from build123d import *

# Parameters (mm, degrees)
SKETCH1_W           = 85.8
SKETCH1_H           = 92.5
SKETCH1_R           = 2.05
BOSS_EXTRUDE1_DEPTH = 3.175
SKETCH2_W           = 85.8
SKETCH2_H           = 92.5
SKETCH2_R           = 1.35
SKETCH2_R_2         = 3.35
BOSS_EXTRUDE2_DEPTH = 1.905
BOSS_EXTRUDE3_START = 1
SKETCH2_3_W         = 85.8
SKETCH2_3_H         = 92.5
SKETCH2_3_R         = 1.35
SKETCH2_3_R_2       = 3.35
BOSS_EXTRUDE3_DEPTH = 1
SKETCH3_W           = 85.8
SKETCH3_H           = 92.5
SKETCH3_W_2         = 75.8
SKETCH3_H_2         = 82.5
BOSS_EXTRUDE4_DEPTH = 4.55
SKETCH4_W           = 14
SKETCH4_H           = 6.75
CUT_EXTRUDE1_DEPTH  = 118.864146478
SKETCH5_W           = 10
SKETCH5_H           = 6
CUT_EXTRUDE2_DEPTH  = 118.864146478
BOSS_EXTRUDE5_DEPTH = 3.5
FILLET1_R           = 2.5
FILLET2_R           = 2.5
FILLET3_R           = 2.5
FILLET4_R           = 2.5
FILLET5_R           = 2.5
CUT_EXTRUDE3_DEPTH  = 3.36
CUT_EXTRUDE4_DEPTH  = 75
SKETCH10_W          = 4.501
SKETCH10_H          = 3
BOSS_EXTRUDE6_DEPTH = 5


with BuildPart() as part:
    # Sketch1 → Boss-Extrude1 (new body)
    with BuildSketch(Plane(origin=(0, 0, 0), x_dir=(1, 0, 0), z_dir=(0, 1, 0))):
        with Locations((36.9, 40.25)):
            Rectangle(SKETCH1_W, SKETCH1_H)
        with Locations(Location((2.5, 12.5, 0), (0, 0, 270))):
            Circle(SKETCH1_R, mode=Mode.SUBTRACT)
        with Locations(Location((18.4, 2.5, 0), (0, 0, 270))):
            Circle(SKETCH1_R, mode=Mode.SUBTRACT)
        with Locations(Location((36.9, 2.5, 0), (0, 0, 270))):
            Circle(SKETCH1_R, mode=Mode.SUBTRACT)
        with Locations(Location((55.4, 2.5, 0), (0, 0, 270))):
            Circle(SKETCH1_R, mode=Mode.SUBTRACT)
        with Locations(Location((29.3, 55.1, 0), (0, 0, 270))):
            Circle(SKETCH1_R, mode=Mode.SUBTRACT)
        with Locations(Location((70.8, 74.5, 0), (0, 0, 270))):
            Circle(SKETCH1_R, mode=Mode.SUBTRACT)
    extrude(amount=BOSS_EXTRUDE1_DEPTH)

    # Sketch2 → Boss-Extrude2 (add)
    # profile 1 of 2: a face of its own
    with BuildSketch(Plane(origin=(0, 0, 0), x_dir=(1, 0, 0), z_dir=(0, 1, 0))):
        with Locations((36.9, 40.25)):
            Rectangle(SKETCH2_W, SKETCH2_H)
        with Locations(Location((2.5, 12.5, 0), (0, 0, 270))):
            Circle(SKETCH2_R, mode=Mode.SUBTRACT)
        with Locations(Location((18.4, 2.5, 0), (0, 0, 270))):
            Circle(SKETCH2_R, mode=Mode.SUBTRACT)
        with Locations(Location((36.9, 2.5, 0), (0, 0, 270))):
            Circle(SKETCH2_R, mode=Mode.SUBTRACT)
        with Locations(Location((55.4, 2.5, 0), (0, 0, 270))):
            Circle(SKETCH2_R, mode=Mode.SUBTRACT)
        with Locations(Location((70.8, 74.5, 0), (0, 0, 270))):
            Circle(SKETCH2_R, mode=Mode.SUBTRACT)
        with BuildLine():
            Line((65.8, 74.5), (65.8, 81.5))
            Line((65.8, 81.5), (-1, 81.5))
            Line((-1, 81.5), (-1, 17.5))
            Line((-1, 17.5), (2.5, 17.5))
            ThreePointArc((2.5, 17.5), (7.5, 12.5), (2.5, 7.5))
            Line((2.5, 7.5), (-1, 7.5))
            Line((-1, 7.5), (-1, -1))
            Line((-1, -1), (13.4, -1))
            Line((13.4, -1), (13.4, 2.5))
            ThreePointArc((13.4, 2.5), (18.4, 7.5), (23.4, 2.5))
            Line((23.4, 2.5), (23.4, -1))
            Line((23.4, -1), (31.9, -1))
            Line((31.9, -1), (31.9, 2.5))
            ThreePointArc((31.9, 2.5), (36.9, 7.5), (41.9, 2.5))
            Line((41.9, 2.5), (41.9, -1))
            Line((41.9, -1), (50.4, -1))
            Line((50.4, -1), (50.4, 2.5))
            ThreePointArc((50.4, 2.5), (55.4, 7.5), (60.4, 2.5))
            Line((60.4, 2.5), (60.4, -1))
            Line((60.4, -1), (74.8, -1))
            Line((74.8, -1), (74.8, 69.5))
            Line((74.8, 69.5), (70.8, 69.5))
            ThreePointArc((70.8, 69.5), (67.264466094, 70.964466094), (65.8, 74.5))
        make_face(mode=Mode.SUBTRACT)
    # profile 2 of 2: a face of its own
    with BuildSketch(Plane(origin=(0, 0, 0), x_dir=(1, 0, 0), z_dir=(0, 1, 0))):
        with Locations(Location((29.3, 55.1, 0), (0, 0, 270))):
            Circle(SKETCH2_R_2)
        with Locations(Location((29.3, 55.1, 0), (0, 0, 270))):
            Circle(SKETCH2_R, mode=Mode.SUBTRACT)
    extrude(amount=-BOSS_EXTRUDE2_DEPTH)

    # Sketch2_3 → Boss-Extrude3 (add)
    # profile 1 of 2: a face of its own
    with BuildSketch(Plane(origin=(0, 0, 0), x_dir=(1, 0, 0), z_dir=(0, 1, 0)).offset(BOSS_EXTRUDE3_START)):
        with Locations((36.9, 40.25)):
            Rectangle(SKETCH2_3_W, SKETCH2_3_H)
        with Locations(Location((2.5, 12.5, 0), (0, 0, 270))):
            Circle(SKETCH2_3_R, mode=Mode.SUBTRACT)
        with Locations(Location((18.4, 2.5, 0), (0, 0, 270))):
            Circle(SKETCH2_3_R, mode=Mode.SUBTRACT)
        with Locations(Location((36.9, 2.5, 0), (0, 0, 270))):
            Circle(SKETCH2_3_R, mode=Mode.SUBTRACT)
        with Locations(Location((55.4, 2.5, 0), (0, 0, 270))):
            Circle(SKETCH2_3_R, mode=Mode.SUBTRACT)
        with Locations(Location((70.8, 74.5, 0), (0, 0, 270))):
            Circle(SKETCH2_3_R, mode=Mode.SUBTRACT)
        with BuildLine():
            Line((65.8, 74.5), (65.8, 81.5))
            Line((65.8, 81.5), (-1, 81.5))
            Line((-1, 81.5), (-1, 17.5))
            Line((-1, 17.5), (2.5, 17.5))
            ThreePointArc((2.5, 17.5), (7.5, 12.5), (2.5, 7.5))
            Line((2.5, 7.5), (-1, 7.5))
            Line((-1, 7.5), (-1, -1))
            Line((-1, -1), (13.4, -1))
            Line((13.4, -1), (13.4, 2.5))
            ThreePointArc((13.4, 2.5), (18.4, 7.5), (23.4, 2.5))
            Line((23.4, 2.5), (23.4, -1))
            Line((23.4, -1), (31.9, -1))
            Line((31.9, -1), (31.9, 2.5))
            ThreePointArc((31.9, 2.5), (36.9, 7.5), (41.9, 2.5))
            Line((41.9, 2.5), (41.9, -1))
            Line((41.9, -1), (50.4, -1))
            Line((50.4, -1), (50.4, 2.5))
            ThreePointArc((50.4, 2.5), (55.4, 7.5), (60.4, 2.5))
            Line((60.4, 2.5), (60.4, -1))
            Line((60.4, -1), (74.8, -1))
            Line((74.8, -1), (74.8, 69.5))
            Line((74.8, 69.5), (70.8, 69.5))
            ThreePointArc((70.8, 69.5), (67.264466094, 70.964466094), (65.8, 74.5))
        make_face(mode=Mode.SUBTRACT)
    # profile 2 of 2: a face of its own
    with BuildSketch(Plane(origin=(0, 0, 0), x_dir=(1, 0, 0), z_dir=(0, 1, 0)).offset(BOSS_EXTRUDE3_START)):
        with Locations(Location((29.3, 55.1, 0), (0, 0, 270))):
            Circle(SKETCH2_3_R_2)
        with Locations(Location((29.3, 55.1, 0), (0, 0, 270))):
            Circle(SKETCH2_3_R, mode=Mode.SUBTRACT)
    extrude(amount=-BOSS_EXTRUDE3_DEPTH)

    # Sketch3 → Boss-Extrude4 (add)
    with BuildSketch(Plane(origin=(0, -1.905, 0), x_dir=(-1, 0, 0), z_dir=(0, -1, 0))):
        with Locations((-36.9, 40.25)):
            Rectangle(SKETCH3_W, SKETCH3_H)
        with Locations((-36.9, 40.25)):
            Rectangle(SKETCH3_W_2, SKETCH3_H_2, mode=Mode.SUBTRACT)
    extrude(amount=BOSS_EXTRUDE4_DEPTH)

    # Sketch4 → Cut-Extrude1 (cut, through all)
    with BuildSketch(Plane.XY):
        with Locations((9.15, -6.47)):
            Rectangle(SKETCH4_W, SKETCH4_H)
        with Locations((27.65, -6.47)):
            Rectangle(SKETCH4_W, SKETCH4_H)
        with Locations((46.15, -6.47)):
            Rectangle(SKETCH4_W, SKETCH4_H)
        with Locations((64.65, -6.47)):
            Rectangle(SKETCH4_W, SKETCH4_H)
    extrude(amount=CUT_EXTRUDE1_DEPTH, mode=Mode.SUBTRACT)

    # Sketch5 → Cut-Extrude2 (cut, through all)
    with BuildSketch(Plane.XY):
        with Locations((58, -7.455)):
            Rectangle(SKETCH5_W, SKETCH5_H)
    extrude(amount=-CUT_EXTRUDE2_DEPTH, mode=Mode.SUBTRACT)

    # Sketch6 → Boss-Extrude5 (add)
    with BuildSketch(Plane.ZY.offset(6)):
        with BuildLine():
            Line((-59.6, 0), (-59.6, -8.95))
            Line((-59.6, -8.95), (-59.131128874, -8.95))
            ThreePointArc((-59.131128874, -8.95), (-55.1, -6.45), (-51.068871126, -8.95))
            Line((-51.068871126, -8.95), (-50.6, -8.95))
            Line((-50.6, -8.95), (-50.6, 0))
            Line((-50.6, 0), (-59.6, 0))
        make_face()
    extrude(amount=-BOSS_EXTRUDE5_DEPTH)

    # Fillet1
    fillet1_edges = [part.edges().sort_by_distance(p)[0] for p in [
        (79.8, -1.64, 6),
    ]]
    fillet(fillet1_edges, radius=FILLET1_R)

    # Fillet2
    fillet2_edges = [part.edges().sort_by_distance(p)[0] for p in [
        (79.8, -1.64, -86.5),
    ]]
    fillet(fillet2_edges, radius=FILLET2_R)

    # Fillet3
    fillet3_edges = [part.edges().sort_by_distance(p)[0] for p in [
        (-6, -1.64, -86.5),
    ]]
    fillet(fillet3_edges, radius=FILLET3_R)

    # Fillet4
    fillet4_edges = [part.edges().sort_by_distance(p)[0] for p in [
        (-6, -1.64, 6),
    ]]
    fillet(fillet4_edges, radius=FILLET4_R)

    # Fillet5
    fillet5_edges = [part.edges().sort_by_distance(p)[0] for p in [
        (79.8, 3.175, -40.25),
        (79.067766953, 3.175, 5.267766953),
        (36.9, 3.175, -86.5),
        (79.067766953, 3.175, -85.767766953),
        (-6, 3.175, -40.25),
        (-5.267766953, 3.175, -85.767766953),
        (36.9, 3.175, 6),
        (-5.267766953, 3.175, 5.267766953),
    ]]
    fillet(fillet5_edges, radius=FILLET5_R)

    # Sketch7 → Cut-Extrude3 (cut)
    with BuildSketch(Plane(origin=(0, -6.455, 0), x_dir=(-1, 0, 0), z_dir=(0, -1, 0))):
        Polygon((-2.15, -2.8), (-0.9, -3.5), (-2.15, -4.2), align=None)
        Polygon((-16.15, -2.8), (-17.4, -3.5), (-16.15, -4.2), align=None)
        Polygon((-20.65, -2.8), (-19.4, -3.5), (-20.65, -4.2), align=None)
        Polygon((-34.65, -2.8), (-35.9, -3.5), (-34.65, -4.2), align=None)
        Polygon((-39.15, -2.8), (-39.15, -4.2), (-37.9, -3.5), align=None)
        Polygon((-53.15, -2.8), (-53.15, -4.2), (-54.4, -3.5), align=None)
        Polygon((-57.65, -4.2), (-56.4, -3.5), (-57.65, -2.8), align=None)
        Polygon((-71.65, -2.8), (-72.9, -3.5), (-71.65, -4.2), align=None)
    extrude(amount=-CUT_EXTRUDE3_DEPTH, mode=Mode.SUBTRACT)

    # Sketch8 → Cut-Extrude4 (cut)
    with BuildSketch(Plane(origin=(0, 0, 0), x_dir=(0, 0, -1), z_dir=(1, 0, 0))):
        Polygon((-4.2, -3.15), (-2.8, -3.15), (-3.5, -1.85), align=None)
    extrude(amount=CUT_EXTRUDE4_DEPTH, mode=Mode.SUBTRACT)

    # Sketch10 → Boss-Extrude6 (add)
    with BuildSketch(Plane.XY.offset(6)):
        with Locations((-0.1005, -1.595)):
            Rectangle(SKETCH10_W, SKETCH10_H)
        with Locations((18.3995, -1.595)):
            Rectangle(SKETCH10_W, SKETCH10_H)
        with Locations((36.8995, -1.595)):
            Rectangle(SKETCH10_W, SKETCH10_H)
        with Locations((55.3995, -1.595)):
            Rectangle(SKETCH10_W, SKETCH10_H)
        with Locations((73.9005, -1.595)):
            Rectangle(SKETCH10_W, SKETCH10_H)
    extrude(amount=-BOSS_EXTRUDE6_DEPTH)


solid = part.part
Can you work these out from the model? Positions are in its coordinate system, mm. A direction names the side the tool comes from. Round coordinates to 2 decimals unless told otherwise and drop trailing zeros. Write each loop counter-clockwise with the first axis right and the second up, starting at its lowest first coordinate (ties: lowest second). Pieces come first, ordered by that corner, then holes. Notation, with made-up numbers: M 63,-7.5 L 116,-7.5 A26 cw 116,7.5 Z; hole C 43,72.5 d7. An arc over 180 degrees is marked long. Use a Markdown table: item, result.
Item 1: We'd pull the mould along Z, two halves only. Please class faces 6 (the face through (55.3, -0.9, -7.5)), 7 (the face through (-4, -8, -50.6)), 8 (the face through (58, -4.455, -84)): released by +Z, released by -Z, zero draft, split by the parting line, or undercut.
Found:
| item | result |
|---|---|
| face 6 | undercut |
| face 7 | released by +Z |
| face 8 | zero draft |
Item 2: For pin 1 Ø4 at (y, z) = (1, -56.5) entering from +X; pin 2 Ø3 at (x, y) = (27, -7) entering from +Z; pin 3 Ø0.7 at (x, y) = (-4.5, -7) entering from -Z; pin 4 Ø3.5 at (x, z) = (18.5, 4) entering from -Y (3 decimals), each with a flat end and sliding along its axis, tell me the tip position at first contact or that it passes through.
Found:
| item | result |
|---|---|
| pin 1 | stops at x = 79.8 |
| pin 2 | stops at z = -81.5 |
| pin 3 | stops at z = -59.6 |
| pin 4 | stops at y = -6.455 |
Item 3: I want a section at B-B (z = -12.5). List the corners of the cut face in (x, y) for me (3 decimals).
Found:
| item | result |
|---|---|
| outline | M -6,-6.455 L -1,-6.455 L -1,-1.905 L 1.15,-1.905 L 1.15,1 L 0.45,1 L 0.45,3.175 L -3.5,3.175 A2.5 ccw -6,0.675 Z; M 3.85,-1.905 L 7.5,-1.905 L 7.5,0 L 74.8,0 L 74.8,-6.455 L 79.8,-6.455 L 79.8,0.675 A2.5 ccw 77.3,3.175 L 4.55,3.175 L 4.55,1 L 3.85,1 Z |
Item 4: Which directions (+Z, -Z, +X, -X, +Y, -Y) give clear straight access to the entire face, cutting with the end or side of a thin tool? Please do faces 1 (the face through (-4.27, -7.2, -57.59)), 2 (the face through (73, -1, -69.5)), 3 (the face through (45, -3.095, 2)), 4 (the face through (37, 1, -1)), 5 (the face through (63, -5, -84)).
Found:
| item | result |
|---|---|
| face 1 | +X, -X, -Y |
| face 2 | -Y |
| face 3 | none |
| face 4 | +Y |
| face 5 | +Z, -Z, -Y |
Item 5: I want a section at A-A (x = 29.3). List the corners of the cut face in (y, z) for me (3 decimals).
Found:
| item | result |
|---|---|
| outline | M -6.455,-86.5 L 0.675,-86.5 A2.5 ccw 3.175,-84 L 3.175,-57.15 L 1,-57.15 L 1,-56.45 L -1.905,-56.45 L -1.905,-58.45 L 0,-58.45 L 0,-81.5 L -6.455,-81.5 Z; M -3.095,1 L 0,1 L 0,-51.75 L -1.905,-51.75 L -1.905,-53.75 L 1,-53.75 L 1,-53.05 L 3.175,-53.05 L 3.175,3.5 A2.5 ccw 0.675,6 L -3.095,6 L -3.095,4.17 L -1.85,3.5 L -3.095,2.83 Z |
Item 6: I want a section at D-D (z = -78). List the corners of the cut face in (x, y) for me (3 decimals).
Found:
| item | result |
|---|---|
| outline | M -6,-6.455 L -1,-6.455 L -1,0 L 65.8,0 L 65.8,-1.905 L 74.8,-1.905 L 74.8,-6.455 L 79.8,-6.455 L 79.8,0.675 A2.5 ccw 77.3,3.175 L -3.5,3.175 A2.5 ccw -6,0.675 Z |
Item 7: I want a section at C-C (z = -64). List the corners of the cut face in (x, y) for me (3 decimals), and give its area (3 significant figures).
Found:
| item | result |
|---|---|
| outline | M -6,-6.455 L -1,-6.455 L -1,0 L 74.8,0 L 74.8,-6.455 L 79.8,-6.455 L 79.8,0.675 A2.5 ccw 77.3,3.175 L -3.5,3.175 A2.5 ccw -6,0.675 Z |
| area | 334 mm2 |
Item 8: If I drill on line 1 along X through (y, z) = (-1, -12.5); line 2 along Z through (x, y) = (70.8, -0.15); line 3 along X through (y, z) = (-5, -76), over which ranges is the centre line in solid material (lowest first)? Write a range as [from, to].
Found:
| item | result |
|---|---|
| line 1 | x = [-6, 1.15], [3.85, 7.5], [74.8, 79.8] |
| line 2 | z = [-86.5, -75.85], [-73.15, -69.5], [1, 6] |
| line 3 | x = [-6, -1], [74.8, 79.8] |
